from build123d import *

# Parameters (mm, degrees)
F0_R     = 3
F1_DEPTH = 18
F2_R     = 3.5
F2_R_2   = 3
F3_DEPTH = 7
F4_W     = 11.7
F4_H     = 11.7
F4_R     = 3.5
F5_DEPTH = 10.1


with BuildPart() as f1:
    # F0 (on Top) → F1 (new body)
    with BuildSketch(Plane.XY):
        Circle(F0_R)
    extrude(amount=F1_DEPTH)

    # F2 (on face) → F3 (join)
    with BuildSketch(Plane(origin=(0, 0, 0), x_dir=(1, 0, 0), z_dir=(0, 0, -1))):
        Circle(F2_R)
        Circle(F2_R_2, mode=Mode.SUBTRACT)
        Circle(F2_R_2)
    extrude(amount=F3_DEPTH)

    # F4 (on face) → F5 (join)
    with BuildSketch(Plane(origin=(0, 0, -7), x_dir=(1, 0, 0), z_dir=(0, 0, -1))):
        Rectangle(F4_W, F4_H)
        Circle(F4_R, mode=Mode.SUBTRACT)
        Circle(F4_R)
    extrude(amount=F5_DEPTH)


solid = f1.part
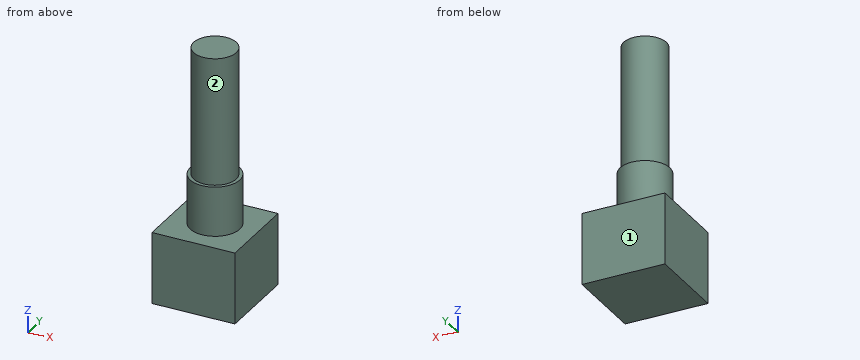
Could you check a few things on this model? Use its own coordinates, in mm. Face numbers are marked on the shaded views. A direction names the side the tool comes from. Coordinates: 2 decimals unless noted, no trailing zeros. Loops run counter-clockwise (first coordinate to the right, second up) from the corner with the lowest first, then second, coordinate; pieces in that order, holes last. Notation, with made-up numbers: (9, 71) -> (33, 71) arc R20 cw to (33, 77) -> close; hole circle Ø4 at (39.5, 55). An arc over 180 degrees is marked (long way). Answer in a Markdown table with one row per item.
(1) For the marked faces 1 and 2, which set-ups out of +Z, -Z, +X, -X, +Y, -Y let a thin tool reach every point of the face, with its end or its side?
Results found:
| item | result |
|---|---|
| face 1 | +Z, -Z, +X, -X, +Y |
| face 2 | +Z |
(2) Will these pins go through, and if not, where does the flat tip stop? pin 1 Ø1 at (x, y) = (-3, -0.5) entering from +Z; pin 2 Ø4 at (y, z) = (3.5, 6) entering from -X; pin 3 Ø4 at (y, z) = (-3, 7) entering from -X; pin 4 Ø2 at (x, z) = (0.5, 7.5) entering from -Y.
Results found:
| item | result |
|---|---|
| pin 1 | stops at z = 18 |
| pin 2 | stops at x = -2.6 |
| pin 3 | stops at x = -2.83 |
| pin 4 | stops at y = -3 |
(3) Imagine slicing it at D-D (x = 4.5). List the corners of the cut face in (y, z) for me.
Results found:
| item | result |
|---|---|
| outline | (-5.85, -17.1) -> (5.85, -17.1) -> (5.85, -7) -> (-5.85, -7) -> close |
(4) Imagine slicing it at A-A (x = 0). List the corners of the cut face in (y, z) for me.
Results found:
| item | result |
|---|---|
| outline | (-5.85, -17.1) -> (5.85, -17.1) -> (5.85, -7) -> (3.5, -7) -> (3.5, 0) -> (3, 0) -> (3, 18) -> (-3, 18) -> (-3, 0) -> (-3.5, 0) -> (-3.5, -7) -> (-5.85, -7) -> close |
(5) If I drill on probe 1 along Z at (x, y) = (3.25, 1); probe 2 along Z at (x, y) = (1.5, -4.5); probe 3 along Y at (x, z) = (0, -3), over which ranges is the centre line in solid material (lowest first)?
Results found:
| item | result |
|---|---|
| probe 1 | z = -17.1 to 0 |
| probe 2 | z = -17.1 to -7 |
| probe 3 | y = -3.5 to 3.5 |
(6) Imagine slicing it at C-C (z = 9). List the corners of the cut face in (x, y) for me.
Results found:
| item | result |
|---|---|
| outline | circle Ø6 at (0, 0) |
